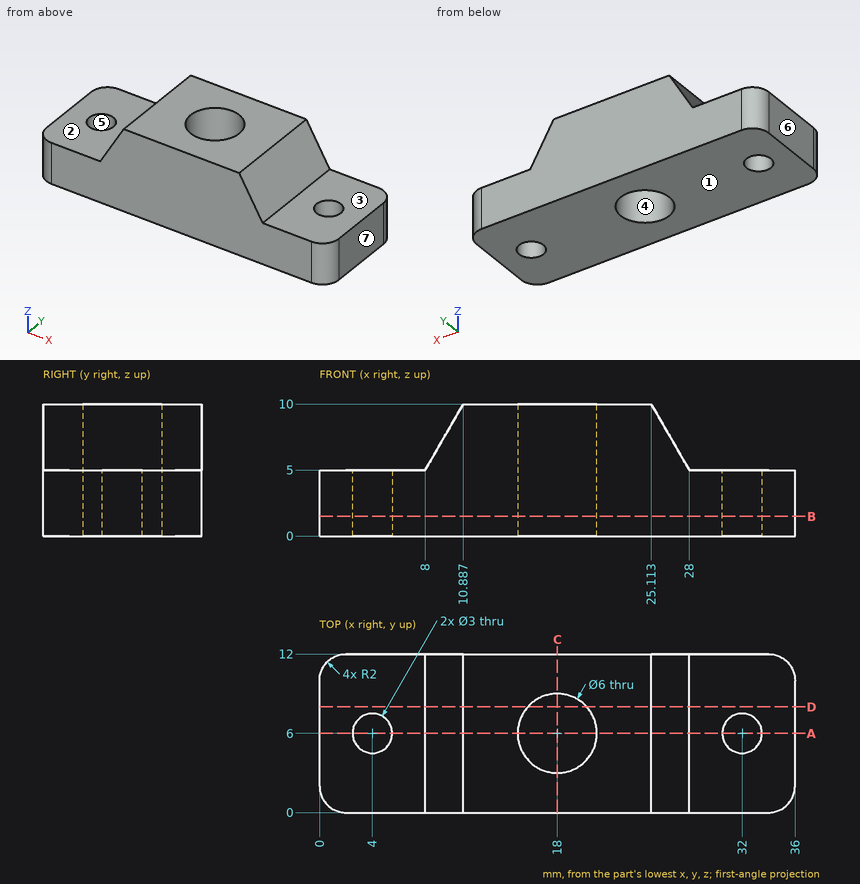
Could you check a few things on this drawing? It's one solid part, dimensions in mm from its lowest x, y, z. A direction names the side the tool comes from. Round coordinates to 2 decimals unless told otherwise and drop trailing zeros. Order: outer loops, then holes, each group sorted by start corner. A loop starts at its lowest first (then second) coordinate and runs counter-clockwise, first axis right, second up.
Q1. Imagine slicing it at C-C, the plane x = 18. List the corners of the cut face in (y, z) for me, then the cut area to 3 significant figures.
Geometry says:
outline: (0, 0) - (3, 0) - (3, 10) - (0, 10) - close; (9, 0) - (12, 0) - (12, 10) - (9, 10) - close
area: 60.0 mm2
Q2. Imagine slicing it at D-D, the plane y = 8. List the corners of the cut face in (x, z) for me.
Geometry says:
outline: (0, 0) - (15.76, 0) - (15.76, 10) - (10.89, 10) - (8, 5) - (0, 5) - close; (20.24, 0) - (36, 0) - (36, 5) - (28, 5) - (25.11, 10) - (20.24, 10) - close
Q3. Please list where these lines run through material, in increasing order: probe 1 along Y at (x, z) = (32, 3); probe 2 along Z at (x, y) = (2, 3.5); probe 3 along Y at (x, z) = (18, 2).
Geometry says:
probe 1: y = 0 to 4.5, 7.5 to 12
probe 2: z = 0 to 5
probe 3: y = 0 to 3, 9 to 12
Q4. Imagine slicing it at A-A, the plane y = 6. List the corners of the cut face in (x, z) for me.
Geometry says:
outline: (0, 0) - (2.5, 0) - (2.5, 5) - (0, 5) - close; (5.5, 0) - (15, 0) - (15, 10) - (10.89, 10) - (8, 5) - (5.5, 5) - close; (21, 0) - (30.5, 0) - (30.5, 5) - (28, 5) - (25.11, 10) - (21, 10) - close; (33.5, 0) - (36, 0) - (36, 5) - (33.5, 5) - close
Q5. I'm going to push flat-ended pins straight in: P1, Ø3, axis at x = 17, y = 7, coming from the +Z side; P2, Ø5, axis at x = 32, y = 6, coming from the +Z side. Where does each tip first touch, or does it pass through?
Geometry says:
P1: passes through
P2: stops at z = 5
Q6. Thinking about a two-plate mould opening in X: for the marked faces 4, 5, 6 and 7, which applies, released by +X, released by -X, zero draft, split by the parting line, or undercut?
Geometry says:
face 4: undercut
face 5: undercut
face 6: released by -X
face 7: released by +X
Q7. Which directions (+Z, -Z, +X, -X, +Y, -Y) give clear straight access to the entire face, cutting with the end or side of a thin tool? Please do the marked faces 1, 2 and 3.
Geometry says:
face 1: -Z, +X, -X, +Y, -Y
face 2: +Z, -X, +Y, -Y
face 3: +Z, +X, +Y, -Y
Q8. Imagine slicing it at B-B, the plane z = 1.5. List the corners of the cut face in (x, y) for me.
Geometry says:
outline: (0, 2) arc R2 ccw to (2, 0) - (34, 0) arc R2 ccw to (36, 2) - (36, 10) arc R2 ccw to (34, 12) - (2, 12) arc R2 ccw to (0, 10) - close; hole circle Ø3 at (4, 6); hole circle Ø6 at (18, 6); hole circle Ø3 at (32, 6)
